Drawing for the job (mm, zero at the part's lowest x, y, z). A direction names the side the tool comes from. Round coordinates to 2 decimals unless told otherwise and drop trailing zeros. Loops run counter-clockwise (first coordinate to the right, second up) from the corner with the lowest first, then second, coordinate; pieces in that order, holes last. Notation, with made-up numbers: (17, 20) - (55, 20) arc R16 ccw to (55, 32) - close; hole circle Ø3 at (66.25, 54.25). An arc over 180 degrees is marked (long way). Put each result on its own line as item: value.
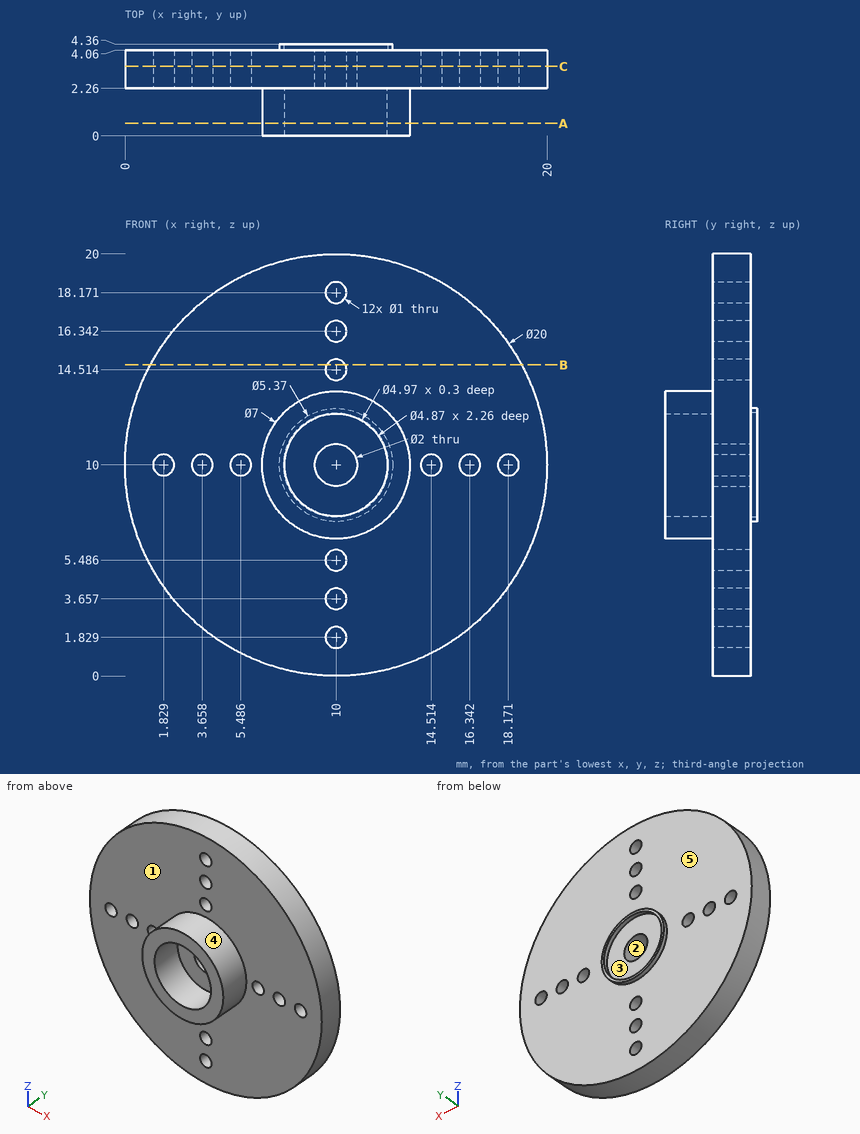
1. Two-plate mould, pull along Z, no slides. Class the marked faces 3, 4 and 5: pulls with the +Z half, pulls with the -Z half, needs draft (parallel to the pull), parting line crosses it, or undercut.
A:
face 3: undercut
face 4: parting line crosses it
face 5: needs draft
2. Tool access for the marked faces 1 and 2: list every direction of +Z, -Z, +X, -X, +Y, -Y with a clear straight run to the whole face (end or side of a thin tool).
A:
face 1: -Y
face 2: +Y, -Y
3. Pin check, flat tips, straight feed: P1, Ø2, axis at y = 2, z = 12.5, coming from the -X side; P2, Ø3, axis at x = 9.5, z = 4, coming from the +Y side; P3, Ø5, axis at x = 3, z = 8.5, coming from the -Y side. Stop position of each tip, or through.
A:
P1: stops at x = 0.12
P2: stops at y = 4.06
P3: stops at y = 2.26
4. Band-saw the part on C-C (y = 3.3). Give the number of separate pieces and of enclosed holes in the cut face.
A:
separate pieces: 1
enclosed holes: 13
5. Band-saw the part on B-B (z = 14.75). List the corners of the cut face in (x, y).
A:
outline: (1.2, 2.26) - (9.56, 2.26) - (9.56, 4.06) - (1.2, 4.06) - close; (10.44, 2.26) - (18.8, 2.26) - (18.8, 4.06) - (10.44, 4.06) - close
6. Probe line 1 along Y through (x, z) = (15, 5); line 2 along Z through (x, y) = (9.75, 0.85); line 3 along X through (y, z) = (3.3, 4) (1 decimal). List the from-to ranges inside material, lowest first. Write a range as [from, to].
A:
line 1: y = [2.26, 4.06]
line 2: z = [6.51, 7.58], [12.42, 13.49]
line 3: x = [2, 9.6], [10.4, 18]
7. Band-saw the part on A-A (y = 0.6). List the corners of the cut face in (x, z) (1 decimal).
A:
outline: circle Ø7 at (10, 10); hole circle Ø4.9 at (10, 10)
